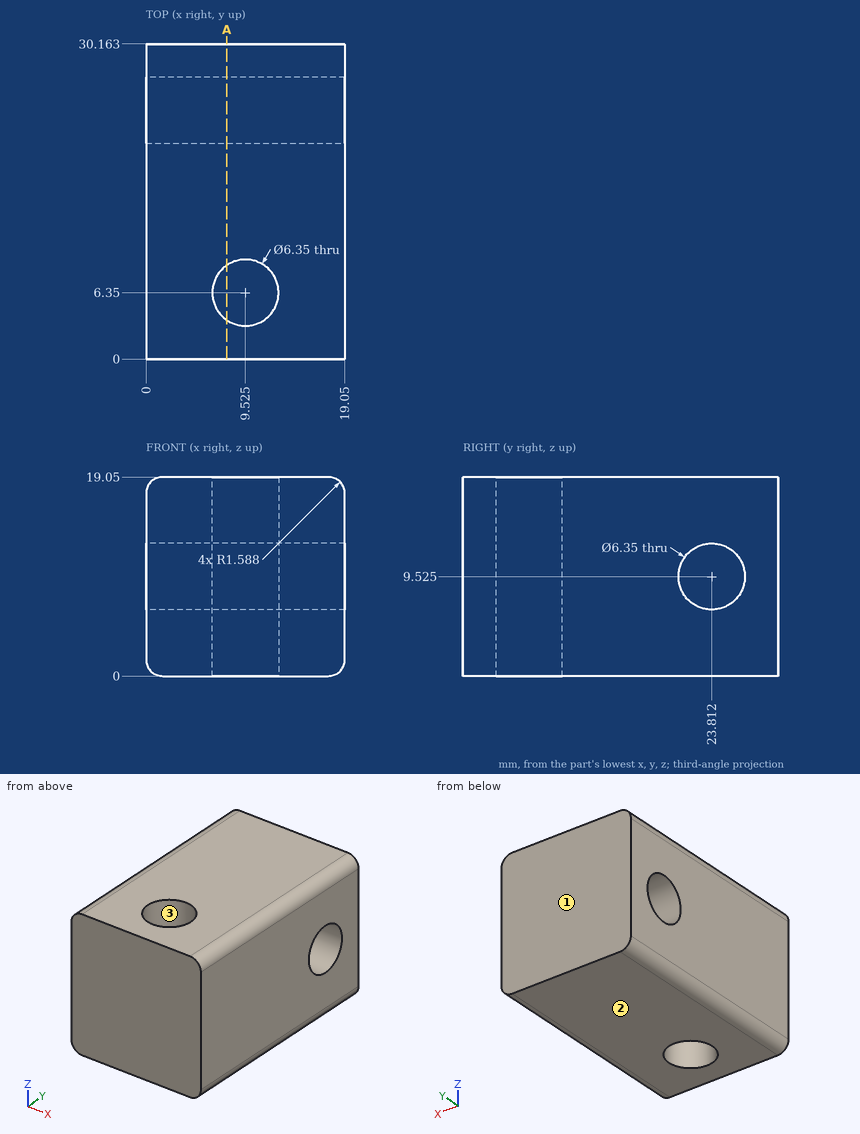
Answer from the drawing. Dimensions are ordinates in mm from the lowest x, y and z of the part. Give positions to 0.01 mm unless a question says otherwise; leave off trailing zeros.
Item 1: The part is cut by section A-A (x = 7.75). Give the number of separate pieces and of enclosed holes in the cut face.
Item 2: Find the intervals of material crossed by line 1 along Z through (x, y) = (1.5, 24) (1 decimal); line 2 along Y through (x, z) = (13.5, 9.75) (1 decimal); line 3 along Y through (x, z) = (11.5, 13.25) (1 decimal), in increasing order.
Item 3: The mould has two halves that part along Y. Classify the marked faces 1, 2 and 3: released by +Y, released by -Y, zero draft, split by the parting line, or undercut.
Taken from the geometry:
1. separate pieces: 2
1. enclosed holes: 1
2. line 1: z = 0 to 6.4, 12.7 to 19
2. line 2: y = 0 to 20.6, 27 to 30.2
2. line 3: y = 0 to 3.9, 8.8 to 30.2
3. face 1: released by +Y
3. face 2: zero draft
3. face 3: undercut
